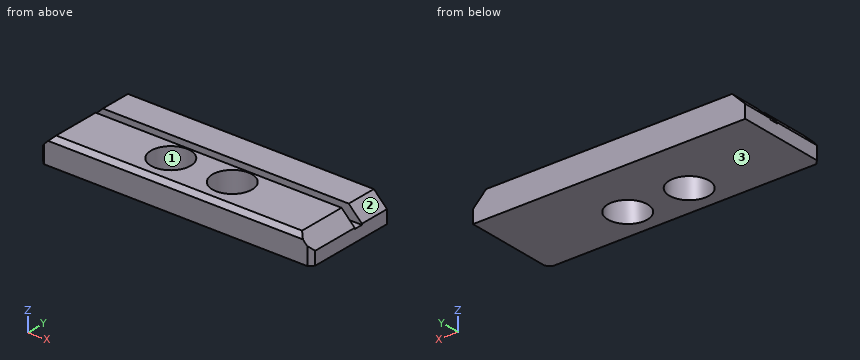
from build123d import *

# Parameters (mm, degrees)
SKETCH1_W          = 393.7
SKETCH1_H          = 38.1
EXTRUDE1_DEPTH     = 133.35
CHAMFER1_SIZE      = 19.05
CHAMFER2_SIZE      = 6.35
SKETCH2_R          = 28.575
CUT_EXTRUDE1_DEPTH = 242.945417109
SKETCH3_W          = 406.514857882
SKETCH3_H          = 12.7
CUT_EXTRUDE2_DEPTH = 22.225


with BuildPart() as part:
    # Sketch1 → Extrude1 (new body)
    with BuildSketch(Plane(origin=(0, 1.6002, 0), x_dir=(1, 0, 0), z_dir=(0, 1, 0))):
        with Locations((0, 20.6502)):
            Rectangle(SKETCH1_W, SKETCH1_H)
    extrude(amount=EXTRUDE1_DEPTH)

    # Chamfer1
    chamfer1_edges = [part.edges().sort_by_distance(p)[0] for p in [
        (196.85, 68.2752, -1.6002),
        (-196.85, 68.2752, -1.6002),
    ]]
    chamfer(chamfer1_edges, length=CHAMFER1_SIZE)

    # Chamfer2
    chamfer2_edges = [part.edges().sort_by_distance(p)[0] for p in [
        (196.85, 1.6002, -30.1752),
        (0, 1.6002, -1.6002),
        (-196.85, 1.6002, -30.1752),
    ]]
    chamfer(chamfer2_edges, length=CHAMFER2_SIZE)

    # Sketch2 → Cut-Extrude1 (cut, through all)
    with BuildSketch(Plane.XY):
        with Locations((-44.45, 47.625)):
            Circle(SKETCH2_R)
        with Locations(Location((44.45, 47.625, 0), (0, 0, 180))):
            Circle(SKETCH2_R)
    extrude(amount=-CUT_EXTRUDE1_DEPTH, mode=Mode.SUBTRACT)

    # Sketch3 → Cut-Extrude2 (cut)
    with BuildSketch(Plane.XY):
        with Locations((0, 84.1502)):
            Rectangle(SKETCH3_W, SKETCH3_H)
    extrude(amount=-CUT_EXTRUDE2_DEPTH, mode=Mode.SUBTRACT)


solid = part.part
Part model, mm, in its own coordinate system. Face numbers are marked on the shaded views. Coordinates: 2 decimals unless noted, no trailing zeros. Loops run counter-clockwise (first coordinate to the right, second up) from the corner with the lowest first, then second, coordinate; pieces in that order, holes last. Notation, with made-up numbers: M 60.5,-18 L 81.5,-18 A21 cw 81.5,10 Z; hole C -23,35 d3. An arc over 180 degrees is marked long. Use a Markdown table: item, result. Add a question column.
Q1. Mould opens along X. For the marked faces 1, 2 and 3 say: +X half, -X half, draft (parallel to the pull), parting line (faces both ways), or undercut.
Q2. Cut at C-C (x = 139.5). Write the cut outline in (y, z) (3 decimals), and give its area (3 significant figures).
Q3. Cut at D-D (y = 15). Write the cut outline in (x, z).
Q4. Cut at A-A (x = 44.45). Write the cut outline in (y, z) (3 decimals), and give its area (3 significant figures).
Q5. Pin check, flat tips, straight feed: P1, Ø8, axis at x = -60, y = 67.5, coming from the +Z side; P2, Ø4, axis at x = 38, y = 84, coming from the +Z side (3 decimals). Stop position of each tip, or through.
Q6. Cut at B-B (y = 39.5). Write the cut outline in (x, z).
Q7. Probe L1, parallel to Y at x = 44, z = -22; L2, parallel to X at y = 48, z = -32.5; L3, parallel to Y at x = 44.45, z = -24.5. List the from-to ranges inside material, lowest first.
Worked out:
| question | item | result |
|---|---|---|
| 1 | face 1 | undercut |
| 1 | face 2 | +X half |
| 1 | face 3 | draft |
| 2 | outline | M 1.6,-39.7 L 134.95,-39.7 L 134.95,-1.6 L 90.5,-1.6 L 90.5,-22.225 L 77.8,-22.225 L 77.8,-1.6 L 7.95,-1.6 L 1.6,-7.95 Z |
| 2 | area | 4,800 mm2 |
| 3 | outline | M -196.85,-39.7 L 196.85,-39.7 L 196.85,-20.65 L 177.8,-1.6 L -177.8,-1.6 L -196.85,-20.65 Z |
| 4 | outline | M 1.6,-39.7 L 19.05,-39.7 L 19.05,-1.6 L 7.95,-1.6 L 1.6,-7.95 Z; M 76.2,-39.7 L 134.95,-39.7 L 134.95,-1.6 L 90.5,-1.6 L 90.5,-22.225 L 77.8,-22.225 L 77.8,-1.6 L 76.2,-1.6 Z |
| 4 | area | 2,620 mm2 |
| 5 | P1 | stops at z = -1.6 |
| 5 | P2 | stops at z = -22.225 |
| 6 | outline | M -196.85,-39.7 L -71.85,-39.7 L -71.85,-1.6 L -177.8,-1.6 L -196.85,-20.65 Z; M -17.05,-39.7 L 17.05,-39.7 L 17.05,-1.6 L -17.05,-1.6 Z; M 71.85,-39.7 L 196.85,-39.7 L 196.85,-20.65 L 177.8,-1.6 L 71.85,-1.6 Z |
| 7 | L1 | y = 1.6 to 19.05, 76.2 to 77.8, 90.5 to 134.95 |
| 7 | L2 | x = -196.85 to -73.02, -15.88 to 15.88, 73.02 to 196.85 |
| 7 | L3 | y = 1.6 to 19.05, 76.2 to 134.95 |
